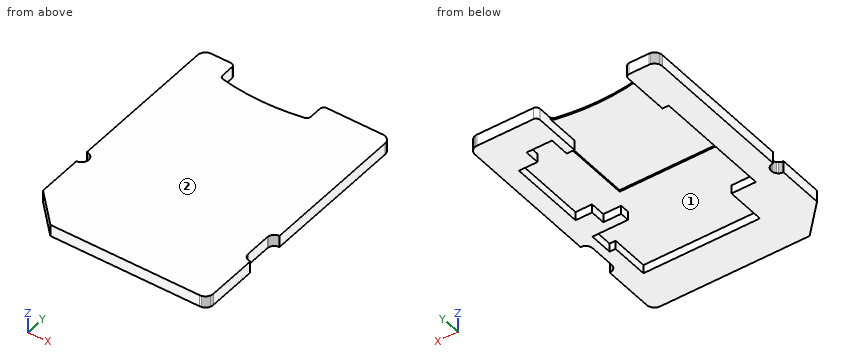
```python
from build123d import *

# Parameters (mm, degrees)
AUFSATZ_LINEAR_START            = 0.1
AUFSATZ_LINEAR_AUSTRAGEN1_DEPTH = 1.5
SCHNITT_LINEAR_AUSTRAGEN1_DEPTH = 1.2
SKIZZE3_W                       = 13.0432381
SKIZZE3_H                       = 9.22364084
SCHNITT_LINEAR_AUSTRAGEN2_DEPTH = 1.4
SKIZZE4_W                       = 11.271857287
SKIZZE4_H                       = 8.011580578
SCHNITT_LINEAR_AUSTRAGEN3_DEPTH = 1.4
SCHNITT_LINEAR_AUSTRAGEN4_DEPTH = 152.434342208
VERRUNDUNG1_R                   = 0.5
VERRUNDUNG2_R                   = 0.5


with BuildPart() as part:
    # Skizze1 → Aufsatz-Linear austragen1 (new body)
    with BuildSketch(Plane.XY.offset(AUFSATZ_LINEAR_START)):
        Polygon((121.99509, -56.619215), (121.8, -56.6), (99.8, -56.6), (99.60491, -56.619215), (99.417317, -56.676121), (99.24443, -56.768531), (99.092894, -56.892894), (98.968531, -57.04443), (98.876121, -57.217317), (98.819215, -57.40491), (98.8, -57.6), (98.8, -76.95), (98.987121, -76.969667), (99.166063, -77.027809), (99.329007, -77.121885), (99.46883, -77.247782), (99.579423, -77.4), (99.655951, -77.571885), (99.69507, -77.755924), (99.69507, -77.944076), (99.655951, -78.128115), (99.579423, -78.3), (99.46883, -78.452218), (99.329007, -78.578115), (99.166063, -78.672191), (98.987121, -78.730333), (98.8, -78.75), (98.8, -84.6), (102.675, -88.6), (121.8, -88.6), (121.99509, -88.580785), (122.182683, -88.52388), (122.35557, -88.43147), (122.507107, -88.307107), (122.63147, -88.15557), (122.72388, -87.982683), (122.780785, -87.79509), (122.8, -87.6), (122.8, -81.15), (122.599731, -81.127435), (122.409505, -81.060872), (122.238859, -80.953648), (122.096352, -80.811141), (121.989128, -80.640495), (121.922565, -80.450269), (121.9, -80.25), (121.9, -76.95), (121.922565, -76.749731), (121.989128, -76.559505), (122.096352, -76.388859), (122.238859, -76.246352), (122.409505, -76.139128), (122.599731, -76.072565), (122.8, -76.05), (122.8, -57.6), (122.780785, -57.40491), (122.72388, -57.217317), (122.63147, -57.04443), (122.507107, -56.892893), (122.35557, -56.76853), (122.182683, -56.67612), align=None)
    extrude(amount=AUFSATZ_LINEAR_AUSTRAGEN1_DEPTH)

    # Skizze2 → Schnitt-Linear austragen1 (cut)
    with BuildSketch(Plane.XY):
        Polygon((102.017864846, -63.099173962), (102.017864846, -78.324168195), (105.146811161, -78.324168195), (105.146811161, -83.287975006), (120.056496088, -83.287975006), (120.056496088, -78.427117377), (120.827696552, -78.427117377), (120.827696552, -75.425497639), (116.267566255, -75.425497639), (116.267566255, -74.231533011), (118.554332467, -74.231533011), (118.554332467, -72.276257259), (120.6715821, -72.276257259), (120.6715821, -62.401228596), (118.309565205, -62.401228596), (118.309565205, -60.50461088), (115.061102946, -60.50461088), (115.061102946, -63.099173962), align=None)
    extrude(amount=SCHNITT_LINEAR_AUSTRAGEN1_DEPTH, mode=Mode.SUBTRACT)

    # Skizze3 → Schnitt-Linear austragen2 (cut)
    with BuildSketch(Plane.XY):
        with Locations((108.539483896, -67.710994382)):
            Rectangle(SKIZZE3_W, SKIZZE3_H)
    extrude(amount=SCHNITT_LINEAR_AUSTRAGEN2_DEPTH, mode=Mode.SUBTRACT)

    # Skizze4 → Schnitt-Linear austragen3 (cut)
    with BuildSketch(Plane.XY):
        with Locations((108.449834452, -59.786485977)):
            Rectangle(SKIZZE4_W, SKIZZE4_H)
    extrude(amount=SCHNITT_LINEAR_AUSTRAGEN3_DEPTH, mode=Mode.SUBTRACT)

    # Skizze5 → Schnitt-Linear austragen4 (cut, through all)
    with BuildSketch(Plane.XY):
        with BuildLine():
            Line((114.085763095, -56.6), (114.085763095, -59.115588122))
            ThreePointArc((114.085763095, -59.115588122), (108.449834452, -59.703189112), (102.813905808, -59.115588122))
            Line((102.813905808, -59.115588122), (102.813905808, -56.6))
            Line((102.813905808, -56.6), (114.085763095, -56.6))
        make_face()
    extrude(amount=SCHNITT_LINEAR_AUSTRAGEN4_DEPTH, mode=Mode.SUBTRACT)

    # Verrundung1
    verrundung1_edges = [part.edges().sort_by_distance(p)[0] for p in [
        (102.813905808, -56.6, 0.85),
        (114.085763095, -56.6, 0.85),
    ]]
    fillet(verrundung1_edges, radius=VERRUNDUNG1_R)

    # Verrundung2
    verrundung2_edges = [part.edges().sort_by_distance(p)[0] for p in [
        (114.085763095, -59.115588122, 1.5),
        (102.813905808, -59.115588122, 1.5),
    ]]
    fillet(verrundung2_edges, radius=VERRUNDUNG2_R)


solid = part.part
```
Check sheet for the modelled part. Datum: model origin and axes. Units: mm. Face numbers are marked on the shaded views. Coordinates: 2 decimals unless noted, no trailing zeros. Write each loop counter-clockwise with the first axis right and the second up, starting at its lowest first coordinate (ties: lowest second). Pieces come first, ordered by that corner, then holes. Notation, with made-up numbers: M 27.5,25 L 46.5,25 A13 cw 46.5,44 Z; hole C 56.5,65.5 d11. An arc over 180 degrees is marked long. Use one line per item in the form item = value.
Item 1: Gauge pin test, flat ends, axial feed: pin 1 Ø0.6 at (x, z) = (102, 1) entering from -Y; pin 2 Ø5 at (x, y) = (106, -66) entering from -Z. Record the tip position at first contact, or that the pin passes through.
Answer below:
pin_1 = -88.21
pin_2 = 1.4
Item 2: Material ranges on L1, parallel to X at y = -79, z = 0.9; L2, parallel to Y at x = 118.75, z = 0.95; L3, parallel to Y at x = 118.25, z = 0.55, recorded low to high. Write a range as from..to.
Answer below:
L1 = 98.8..105.15, 120.06..121.9
L2 = -88.6..-83.29, -75.43..-72.28, -62.4..-56.6
L3 = -88.6..-83.29, -75.43..-74.23, -60.5..-56.6
Item 3: Sectioned sample at C-C, the plane y = -71. Record the cut outline in (x, z).
Answer below:
outline = M 98.8,0.1 L 102.02,0.1 L 102.02,1.4 L 115.06,1.4 L 115.06,1.2 L 120.67,1.2 L 120.67,0.1 L 122.8,0.1 L 122.8,1.6 L 98.8,1.6 Z
Item 4: Sectioned sample at B-B, the plane y = -79.5. Record the cut outline in (x, z).
Answer below:
outline = M 98.8,0.1 L 105.15,0.1 L 105.15,1.2 L 120.06,1.2 L 120.06,0.1 L 121.9,0.1 L 121.9,1.6 L 98.8,1.6 Z
Item 5: Sectioned sample at A-A, the plane x = 117.5. Record the cut outline in (y, z).
Answer below:
outline = M -88.6,0.1 L -83.29,0.1 L -83.29,1.2 L -75.43,1.2 L -75.43,0.1 L -74.23,0.1 L -74.23,1.2 L -60.5,1.2 L -60.5,0.1 L -56.6,0.1 L -56.6,1.6 L -88.6,1.6 Z
Item 6: Release check for a two-part mould opening along X. For the marked faces 1 and 2 record: pulls with the +X half, pulls with the -X half, needs draft (parallel to the pull), parting line crosses it, or undercut.
Answer below:
face_1 = undercut
face_2 = needs draft
Item 7: Sectioned sample at D-D, the plane x = 106.75. Record the cut outline in (y, z), and give its area (3 significant figures).
Answer below:
outline = M -88.6,0.1 L -83.29,0.1 L -83.29,1.2 L -72.32,1.2 L -72.32,1.4 L -59.65,1.4 L -59.65,1.6 L -88.6,1.6 Z
area = 14.9 mm^2
